from build123d import *

# Parameters (mm, degrees)
F1_DEPTH = 38
F2_R     = 18.99999


# Not quite as in the source:
# - a fillet or chamfer is up to 0.001 mm smaller than in the source, because OpenCascade refuses the exact size


with BuildPart() as f1:
    # F0 (on Front) → F1 (new body)
    with BuildSketch(Plane.XZ):
        Polygon((-19.9589891719, 57), (-33.4447937101, 57), (-33.4447937101, 13.7555195992), (-33.4447937101, 0), (-19.9589891719, 0), (23.5552062899, 0), (23.5552062899, 13.7555195992), (-19.9589891719, 13.7555195992), align=None)
    extrude(amount=F1_DEPTH)

    # F2 (radius 19 in the source; OpenCascade refuses exactly that, so slightly less here)
    f2_edges = [f1.edges().sort_by_distance(p)[0] for p in [
        (-26.701891, -38, 57),
        (-26.701891, 0, 57),
        (23.555206, 0, 6.87776),
        (23.555206, -38, 6.87776),
    ]]
    fillet(f2_edges, radius=F2_R)


solid = f1.part
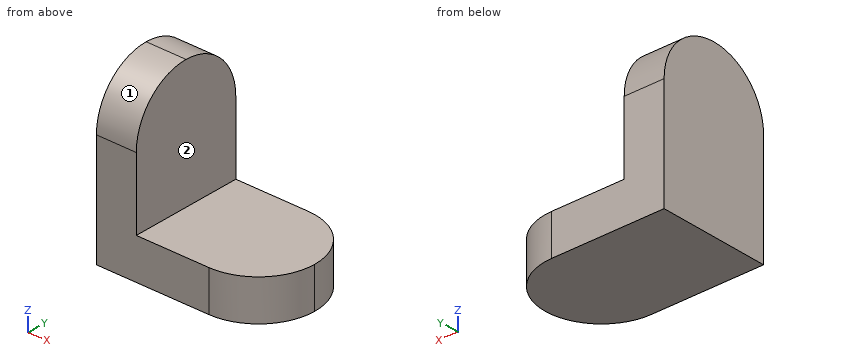
Build history of the part. All positions in model axes, mm. Face numbers are marked on the shaded views. A direction names the side the tool comes from. Round coordinates to 2 decimals unless told otherwise and drop trailing zeros. Loops run counter-clockwise (first coordinate to the right, second up) from the corner with the lowest first, then second, coordinate; pieces in that order, holes last. Notation, with made-up numbers: (32.5, 84) -> (43.5, 84) arc R11 cw to (43.5, 96) -> close; hole circle Ø8 at (-30, 38). An arc over 180 degrees is marked (long way). Use CSV: the item, a comma, the result in double quotes. Start each with the question number.
Q1. Saw through at C-C on z = 53.5. Give the cut face in (x, y).
Q2. Drill centre lines: L1, parallel to X at y = -31.5, z = 21.5; L2, parallel to Z at x = -1, y = -24; L3, parallel to Z at x = -26.5, y = -6. Where is each one in solid material? Low to high.
Q3. Which spindle directions (+Z, -Z, +X, -X, +Y, -Y) get a long thin tool onto all of the face, cutting with end or side? Do the marked faces 1 and 2. Say none if no direction does.
Q4. Saw through at B-B on y = -17.5. Give the cut face in (x, z).
Q5. Saw through at A-A on x = -4. Give the cut face in (y, z).
Q6. Flat gauge pins, fed straight in: pin 1 Ø8 at (x, z) = (17.5, 10.5) entering from +Y; pin 2 Ø1.5 at (x, y) = (3, -7.5) entering from +Z. Where does each tip first touch, or does it go through?
Solutions:
1,outline,"(-33.44, -29.99) -> (-19.96, -29.99) -> (-19.96, -8.01) -> (-33.44, -8.01) -> close"
2,L1,"x = -33.44 to -19.96"
2,L2,"z = 0 to 13.76"
2,L3,"z = 0 to 51.86"
3,face 1,"+Z, +X, -X, -Y"
3,face 2,"+Z, +X, +Y, -Y"
4,outline,"(-33.44, 0) -> (23.5, 0) -> (23.5, 13.76) -> (-19.96, 13.76) -> (-19.96, 56.94) -> (-33.44, 56.94) -> close"
5,outline,"(-38, 0) -> (0, 0) -> (0, 13.76) -> (-38, 13.76) -> close"
6,pin 1,"stops at y = -2.24"
6,pin 2,"stops at z = 13.76"
